Model file for the job. Use its own axes, mm. A direction names the side the tool comes from. Round coordinates to 2 decimals unless told otherwise and drop trailing zeros. Write each loop counter-clockwise with the first axis right and the second up, starting at its lowest first coordinate (ties: lowest second). Pieces come first, ordered by that corner, then holes.
Autodesk Inventor part; units mm, degrees
ref_plane "YZ Plane" through (0, 0, 0) normal (1, 0, 0) x (0, 1, 0)
ref_plane "XZ Plane" through (0, 0, 0) normal (0, 1, 0) x (-1, 0, 0)
ref_plane "XY Plane" through (0, 0, 0) normal (0, 0, 1) x (1, 0, 0)
sketch "Esboço1" plane through (0, 0, 0) normal (0, 0, 1) x (1, 0, 0)
  line L0 (0, 12.7) -> (125, 12.7)
  line L1 (125, 12.7) -> (125, -39.3)
  line L2 (125, -39.3) -> (0, -39.3)
  line L3 (0, -39.3) -> (0, 12.7)
  circle A0 centre (62.5, -20) radius 11.5
  dimension "d0" = 52
  dimension "d1" = 23
  dimension "d2" = 125
extrude "Extrusão1" add sketch "Esboço1" along normal blind 12.7
sketch "Esboço3" plane through (0, 0, 12.7) normal (0, 0, 1) x (1, 0, 0)
  circle A0 centre (75.935, -33.435) radius 2.75 construction
  circle A1 centre (49.065, -33.435) radius 2.75 construction
  circle A2 centre (81.5, -20) radius 2.75 construction
  circle A3 centre (43.5, -20) radius 2.75 construction
  circle A4 centre (49.065, -6.565) radius 2.75 construction
  circle A5 centre (75.935, -6.565) radius 2.75 construction
  point P0 (0, 0)
hole "Furo2" at (75.935, -33.435, 12.7) at (49.065, -33.435, 12.7) at (81.5, -20, 12.7) at (43.5, -20, 12.7) at (49.065, -6.565, 12.7) at (75.935, -6.565, 12.7) direction (0, 0, -1) diameter 4.134 end through all
sketch "Esboço5" plane through (0, 0, 12.7) normal (0, 0, 1) x (1, 0, 0)
  circle A0 centre (6.5, 6.35) radius 2.067
  circle A1 centre (34.5, 6.35) radius 2.067
  circle A2 centre (62.5, 6.35) radius 2.067
  circle A3 centre (90.5, 6.35) radius 2.067
  circle A4 centre (118.5, 6.35) radius 2.067
  point P0 (0, 0)
hole "Furo3" at (6.5, 6.35, 12.7) at (34.5, 6.35, 12.7) at (62.5, 6.35, 12.7) at (90.5, 6.35, 12.7) at (118.5, 6.35, 12.7) direction (0, 0, -1) diameter 5.5 end through all counterbore diameter 8 counterbore depth 6
properties part number "CHAPA_APOIO_CASTANHA_EIXO_Z"
1) Pull direction Y, two halves, no side cores. Call faces 3 (the face through (62, 12.7, 6)), 4 (the face through (62, -7, 12.7)), 5 (the face through (42.88, -21.97, 6.26)): released by +Y, released by -Y, zero draft, split by the parting line, or undercut.
2) Which spindle directions (+Z, -Z, +X, -X, +Y, -Y) get a long thin tool onto all of the face, cutting with end or side? Do faces 1 (the face through (77.953, -32.987, 6.261)), 2 (the face through (114.534, 6.871, 9.658)). Say none if no direction does.
3) Cut at D-D on y = -14. List the corners of the cut face in (x, z), and give its area (3 significant figures).
4) Cut at C-C on x = 62.5. List the corners of the cut face in (y, z), and give its area (3 significant figures).
5) Flat gauge pin, fed straight in: pin 1 Ø7 at (x, y) = (34.5, 6.35) entering from +Z. Where does the tip first touch, or does it go through?
6) Cut at A-A on x = 34.5. List the corners of the cut face in (y, z).
7) Cut at B-B on y = -20. List the corners of the cut face in (x, z).
8) Wall check: probe 1 along X at (y, z) = (6.35, 4.5); probe 2 along Y at (x, z) = (62.5, 2); probe 3 along X at (y, z) = (-6.5, 9.5). Give the ranges that are in metal, low to high.
Result sheet:
1. face 3: released by +Y
1. face 4: zero draft
1. face 5: undercut
2. face 1: +Z, -Z
2. face 2: +Z
3. outline: (0, 0) - (52.69, 0) - (52.69, 12.7) - (0, 12.7) - close; (72.31, 0) - (125, 0) - (125, 12.7) - (72.31, 12.7) - close
3. area: 1,340 mm2
4. outline: (-39.3, 0) - (-31.5, 0) - (-31.5, 12.7) - (-39.3, 12.7) - close; (-8.5, 0) - (3.6, 0) - (3.6, 6.7) - (2.35, 6.7) - (2.35, 12.7) - (-8.5, 12.7) - close; (9.1, 0) - (12.7, 0) - (12.7, 12.7) - (10.35, 12.7) - (10.35, 6.7) - (9.1, 6.7) - close
4. area: 283 mm2
5. pin 1: stops at z = 6.7
6. outline: (-39.3, 0) - (3.6, 0) - (3.6, 6.7) - (2.35, 6.7) - (2.35, 12.7) - (-39.3, 12.7) - close; (9.1, 0) - (12.7, 0) - (12.7, 12.7) - (10.35, 12.7) - (10.35, 6.7) - (9.1, 6.7) - close
7. outline: (0, 0) - (41.43, 0) - (41.43, 12.7) - (0, 12.7) - close; (45.57, 0) - (51, 0) - (51, 12.7) - (45.57, 12.7) - close; (74, 0) - (79.43, 0) - (79.43, 12.7) - (74, 12.7) - close; (83.57, 0) - (125, 0) - (125, 12.7) - (83.57, 12.7) - close
8. probe 1: x = 0 to 3.75, 9.25 to 31.75, 37.25 to 59.75, 65.25 to 87.75, 93.25 to 115.75, 121.25 to 125
8. probe 2: y = -39.3 to -31.5, -8.5 to 3.6, 9.1 to 12.7
8. probe 3: x = 0 to 47, 51.13 to 73.87, 78 to 125
